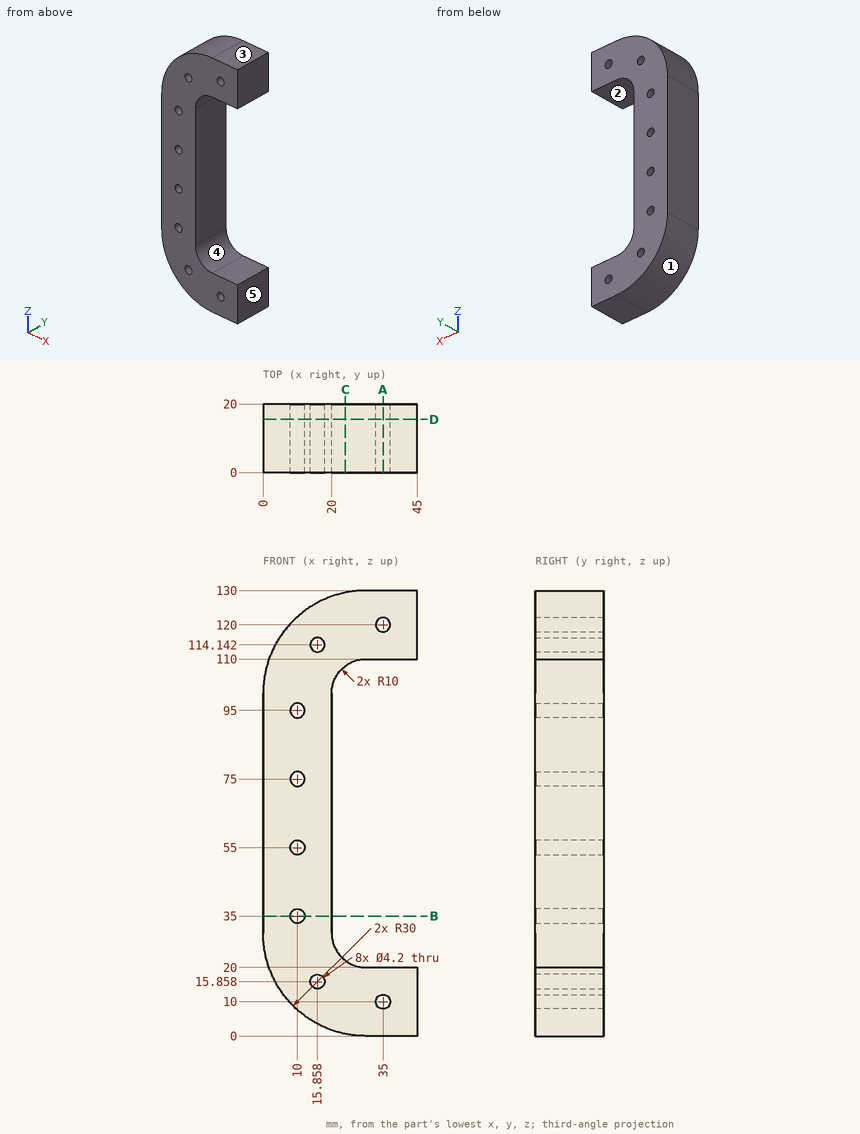
Study the drawing (mm; zero at the part's minimum x, y, z) and answer. A direction names the side the tool comes from. Give positions to 0.01 mm unless a question says otherwise; leave off trailing zeros. Write each loop counter-clockwise with the first axis right and the second up, starting at its lowest first coordinate (ties: lowest second). Pieces come first, ordered by that corner, then holes. Notation, with made-up numbers: (75, -1) -> (95, -1) arc R8 ccw to (95, 10) -> close; hole circle Ø10 at (67, 1.25). An arc over 180 degrees is marked (long way). Answer as a JSON object with one key per item and string values. Group by question number.
1) Find section C-C (x = 24). Write down the section's boundary in (y, z), and give its area (3 significant figures).
2) Find section D-D (y = 15.5). Count the separate pieces of the cut face and the enclosed holes in it, and give its area (3 significant figures).
3) Find section A-A (x = 35). Write down the section's boundary in (y, z).
4) Consider L1, parallel to Z at x = 35, y = 5; L2, parallel to Z at x = 39.5, y = 14; L3, parallel to Z at x = 9.5, y = 16.5. Determine where each line is inside the solid, lowest interval first. Write a range as from..to.
5) The mould has two halves that part along Z. Classify the marked faces 3, 4 and 5: +Z half, -Z half, draft (parallel to the pull), parting line (faces both ways), or undercut.
6) A tool of negligible diameter and unlimited length cuts with its end or side. For the marked faces 1 and 2, from which of +Z, -Z, +X, -X, +Y, -Y can it reach the whole face along a straight path? Write none if from no direction.
7) Each of these flat-tipped pins is pushed along its axis until it touches: P1, Ø3.5, axis at x = 15.86, z = 114.14, coming from the -Y side; P2, Ø3, axis at x = 24.5, y = 12.5, coming from the +Z side. Where does it stop, or does it pass through?
8) Find section B-B (z = 35). Write down the section's boundary in (x, y).
Values follow:
{
 "1": {"outline": "(0, 0.61) -> (20, 0.61) -> (20, 22) -> (0, 22) -> close; (0, 108) -> (20, 108) -> (20, 129.39) -> (0, 129.39) -> close", "area": "856 mm2"},
 "2": {"separate pieces": "1", "enclosed holes": "8", "area": "3,150 mm2"},
 "3": {"outline": "(0, 0) -> (20, 0) -> (20, 7.9) -> (0, 7.9) -> close; (0, 12.1) -> (20, 12.1) -> (20, 20) -> (0, 20) -> close; (0, 110) -> (20, 110) -> (20, 117.9) -> (0, 117.9) -> close; (0, 122.1) -> (20, 122.1) -> (20, 130) -> (0, 130) -> close"},
 "4": {"L1": "z = 0..7.9, 12.1..20, 110..117.9, 122.1..130", "L2": "z = 0..20, 110..130", "L3": "z = 8.1..32.96, 37.04..52.96, 57.04..72.96, 77.04..92.96, 97.04..121.9"},
 "5": {"face 3": "+Z half", "face 4": "undercut", "face 5": "draft"},
 "6": {"face 1": "-Z, -X, +Y, -Y", "face 2": "+X, +Y, -Y"},
 "7": {"P1": "passes through", "P2": "stops at z = 129.73"},
 "8": {"outline": "(0, 0) -> (7.9, 0) -> (7.9, 20) -> (0, 20) -> close; (12.1, 0) -> (20, 0) -> (20, 20) -> (12.1, 20) -> close"}
}
